Part model, mm, in its own coordinate system. A direction names the side the tool comes from. Round coordinates to 2 decimals unless told otherwise and drop trailing zeros. Order: outer loops, then holes, each group sorted by start corner. A loop starts at its lowest first (then second) coordinate and runs counter-clockwise, first axis right, second up. Notation, with made-up numbers: M 16.25,-0.75 L 36.25,-0.75 A22 ccw 36.25,14.25 Z; hole C 77.25,-3.75 d6. An arc over 180 degrees is marked long. Write each question's results on one line, items separated by ' | '. Start each with the question number.
1. Which spindle directions (+Z, -Z, +X, -X, +Y, -Y) get a long thin tool onto all of the face, cutting with end or side? Do faces 4 (the face through (-1, 2, 192)), 5 (the face through (-2, 0, 25)), 6 (the face through (0, 1.5, 225)), 7 (the face through (0.54, -2.44, 200.13)). Say none if no direction does.
2. Drop flat-ended pins along their axis: pin 1 Ø1.8 at (x, y) = (-1, 0) entering from -Z; pin 2 Ø1.5 at (x, z) = (1, 143.5) entering from +Y; pin 3 Ø2 at (x, z) = (0, 226) entering from +Y; pin 4 Ø1 at (x, z) = (-1, 204.5) entering from +Y. Give the stop position or say it passes through.
3. Two-plate mould, pull along Z, no slides. Class faces 1 (the face through (-1, 2, 209.5)), 2 (the face through (0.54, -2.44, 219.61)), 3 (the face through (0, 0, 230)): +Z half, -Z half, draft (parallel to the pull), parting line (faces both ways), or undercut.
4. Probe L1, parallel to Z at x = -1.35, y = -1.8; L2, parallel to Z at x = 0.25, y = 1.4; L3, parallel to Y at x = -1.2, z = 75.5. List the from-to ranges inside material, lowest first. Write a range as [from, to].
5. Band-saw the part on A-A, the plane z = 57.5. List the corners of the cut face in (x, y), then the cut area to 3 significant figures.
```python
from build123d import *

# Parameters (mm, degrees)
SKETCH_1_R           = 2.75
EXTRUDE_6_DEPTH      = 250
SKETCH_22_R          = 3.543321461
SKETCH_22_R_2        = 1.75
CUT_EXTRUDE_16_DEPTH = 25
SKETCH_23_R          = 4.906655543
SKETCH_23_R_2        = 2.5
CUT_EXTRUDE_17_DEPTH = 61
SKETCH_29_R          = 7.224487221
CUT_EXTRUDE_18_DEPTH = 10
CUT_EXTRUDE_19_DEPTH = 20
SKETCH_33_R          = 3.493195313
SKETCH_33_R_2        = 2.5
CUT_EXTRUDE_20_DEPTH = 5
SKETCH_34_R          = 3.783708721
SKETCH_34_R_2        = 1.5
CUT_EXTRUDE_21_DEPTH = 21.5
SKETCH_36_R          = 3.547380577
SKETCH_36_R_2        = 1
CUT_EXTRUDE_22_DEPTH = 1
SKETCH_37_R          = 5.022204732
SKETCH_37_R_2        = 2
CUT_EXTRUDE_23_DEPTH = 1
SKETCH_38_R          = 5.160137664
SKETCH_38_R_2        = 2
CUT_EXTRUDE_24_DEPTH = 1
SKETCH_39_R          = 4.465898571
CUT_EXTRUDE_25_DEPTH = 10


with BuildPart() as part:
    # 草图1 → 凸台-拉伸6 (new body)
    with BuildSketch(Plane.XY):
        Circle(SKETCH_1_R)
    extrude(amount=EXTRUDE_6_DEPTH)

    # 草图22 → 切除-拉伸16 (cut)
    with BuildSketch(Plane(origin=(0, 0, 0), x_dir=(-1, 0, 0), z_dir=(0, 0, -1))):
        Circle(SKETCH_22_R)
        Circle(SKETCH_22_R_2, mode=Mode.SUBTRACT)
    extrude(amount=-CUT_EXTRUDE_16_DEPTH, mode=Mode.SUBTRACT)

    # 草图23 → 切除-拉伸17 (cut, through all)
    with BuildSketch(Plane(origin=(0, 0, 190), x_dir=(-1, 0, 0), z_dir=(0, 0, -1))):
        Circle(SKETCH_23_R)
        Circle(SKETCH_23_R_2, mode=Mode.SUBTRACT)
    extrude(amount=-CUT_EXTRUDE_17_DEPTH, mode=Mode.SUBTRACT)

    # 草图29 → 切除-拉伸18 (cut)
    with BuildSketch(Plane.XY.offset(250)):
        Circle(SKETCH_29_R)
    extrude(amount=-CUT_EXTRUDE_18_DEPTH, mode=Mode.SUBTRACT)

    # 草图32 → 切除-拉伸19 (cut)
    with BuildSketch(Plane.XY.offset(240)):
        with BuildLine():
            Line((-2, 1.5), (2, 1.5))
            ThreePointArc((2, 1.5), (0, 2.5), (-2, 1.5))
        make_face()
    extrude(amount=-CUT_EXTRUDE_19_DEPTH, mode=Mode.SUBTRACT)

    # 草图33 → 切除-拉伸20 (cut)
    with BuildSketch(Plane.XY.offset(190)):
        Circle(SKETCH_33_R)
        Circle(SKETCH_33_R_2, mode=Mode.SUBTRACT)
    extrude(amount=-CUT_EXTRUDE_20_DEPTH, mode=Mode.SUBTRACT)

    # 草图34 → 切除-拉伸21 (cut)
    with BuildSketch(Plane(origin=(0, 0, 0), x_dir=(-1, 0, 0), z_dir=(0, 0, -1))):
        Circle(SKETCH_34_R)
        Circle(SKETCH_34_R_2, mode=Mode.SUBTRACT)
    extrude(amount=-CUT_EXTRUDE_21_DEPTH, mode=Mode.SUBTRACT)

    # 草图36 → 切除-拉伸22 (cut)
    with BuildSketch(Plane(origin=(0, 0, 5), x_dir=(-1, 0, 0), z_dir=(0, 0, -1))):
        Circle(SKETCH_36_R)
        Circle(SKETCH_36_R_2, mode=Mode.SUBTRACT)
    extrude(amount=CUT_EXTRUDE_22_DEPTH, mode=Mode.SUBTRACT)

    # 草图37 → 切除-拉伸23 (cut)
    with BuildSketch(Plane.XY.offset(191)):
        Circle(SKETCH_37_R)
        Circle(SKETCH_37_R_2, mode=Mode.SUBTRACT)
    extrude(amount=CUT_EXTRUDE_23_DEPTH, mode=Mode.SUBTRACT)

    # 草图38 → 切除-拉伸24 (cut)
    with BuildSketch(Plane.XY.offset(208.5)):
        Circle(SKETCH_38_R)
        Circle(SKETCH_38_R_2, mode=Mode.SUBTRACT)
    extrude(amount=CUT_EXTRUDE_24_DEPTH, mode=Mode.SUBTRACT)

    # 草图39 → 切除-拉伸25 (cut)
    with BuildSketch(Plane.XY.offset(240)):
        Circle(SKETCH_39_R)
    extrude(amount=-CUT_EXTRUDE_25_DEPTH, mode=Mode.SUBTRACT)


solid = part.part
```
Solution:
1) face 4: none | face 5: -Z | face 6: +Z, +X, -X, +Y | face 7: +Z
2) pin 1: z = 0 | pin 2: y = 2.74 | pin 3: y = 1.5 | pin 4: y = 2.45
3) face 1: undercut | face 2: draft | face 3: +Z half
4) L1: [25, 191], [192, 208.5], [209.5, 230] | L2: [0, 4], [5, 230] | L3: [-2.47, 2.47]
5) outline: C 0,0 d5.5 | area: 23.8 mm^2
